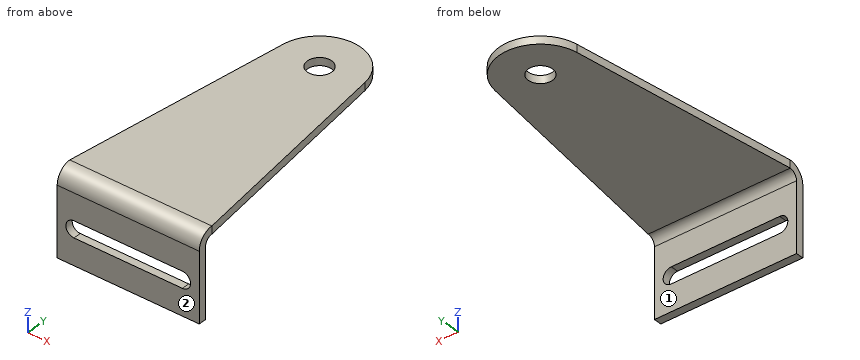
Autodesk Inventor part; units mm, degrees
ref_plane "YZ Plane" through (0, 0, 0) normal (1, 0, 0) x (0, 1, 0)
ref_plane "XZ Plane" through (0, 0, 0) normal (0, 1, 0) x (-1, 0, 0)
ref_plane "XY Plane" through (0, 0, 0) normal (0, 0, 1) x (1, 0, 0)
sketch "Boceto1" plane through (0, 0, 0) normal (0, 1, 0) x (-1, 0, 0)
  line L0 (-17.5, 8.5) -> (17.5, 8.5)
  line L1 (17.5, 8.5) -> (17.5, -8.5)
  line L2 (17.5, -8.5) -> (-17.5, -8.5)
  line L3 (-17.5, -8.5) -> (-17.5, 8.5)
  line L4 (-17.5, 8.5) -> (17.5, -8.5) construction
  line L5 (17.5, 8.5) -> (-17.5, -8.5) construction
  point P0 (0, 0)
  dimension "d0" = 35
  dimension "d1" = 17
extrude "Placa1" add sketch "Boceto1" along normal blind 1.91
sketch "Boceto2" plane through (17.5, 3.82, 10.41) normal (0, 0, 1) x (1, 0, 0)
  line L0 (-35, 0) -> (0, 0)
  line L1 (0, 0) -> (0, 66.18)
  line L2 (0, 66.18) -> (-35, 66.18)
  line L3 (-35, 66.18) -> (-35, 0)
edge flange "Pestaña1" height 70 angle 90 thickness 1.91 bend radius 1.91 thickness toward (0, 0, 1) relief tear relief width 1.91 relief depth 0.955 edges at (0, 1.91, 8.5) wall of the first edge with corners at (-17.5, 3.82, 10.41) (17.5, 3.82, 10.41) (17.5, 70, 10.41) (-17.5, 70, 10.41)
bend "Doblez1"
corner "Esquina1"
sketch "Boceto5" plane through (-17.5, 70, 12.32) normal (0, 0, 1) x (1, 0, 0)
  arc A0 (27.5986, -10.5074) -> (7.4014, -10.5074) centre (17.5, -11.85) ccw
  line L0 (0, -66.18) -> (7.4014, -10.5074)
  line L1 (35, -66.18) -> (27.5986, -10.5074)
  line L2 (0, 0) -> (35, 0)
  line L3 (0, -66.18) -> (0, 0)
  line L4 (0, 0) -> (35, 0)
  line L5 (35, 0) -> (35, -66.18)
  point P0 (17.5, -70)
  dimension "d21" = 20.375
extrude "Cortar2" cut sketch "Boceto5" against normal blind 1.91
sketch "Boceto6" plane through (-17.5, 3.82, 12.32) normal (0, 0, 1) x (1, 0, 0)
  line L0 (7.4014, 55.6726) -> (0, 0)
  line L1 (0, 0) -> (35, 0)
  line L2 (35, 0) -> (27.5986, 55.6726)
  arc A0 (27.5986, 55.6726) -> (7.4014, 55.6726) centre (17.5, 54.33) ccw
  circle A1 centre (17.5, 54.33) radius 3
  point P0 (17.5, -3.82)
  dimension "d26" = 6
extrude "Cortar3" cut sketch "Boceto6" against normal blind 1.91 contours A1
sketch "Boceto7" plane through (0, 1.91, 0) normal (0, 1, 0) x (1, 0, 0)
  line L0 (13.3569, 0) -> (-13.3569, 0) construction
  line L1 (13.3569, 2) -> (-13.3569, 2)
  line L2 (-13.3569, -2) -> (13.3569, -2)
  arc A0 (13.3569, -2) -> (13.3569, 2) centre (13.3569, 0) ccw
  arc A1 (-13.3569, 2) -> (-13.3569, -2) centre (-13.3569, 0) ccw
  point P0 (0, 0)
  dimension "d29" = 4
extrude "Cortar4" cut sketch "Boceto7" against normal blind 1.91
equation "\"d24\" = Grosor"
equation "\"d27\" = Grosor"
equation "\"d30\" = Grosor"
equation "\"d2\" = Grosor"
equation "\"d3\" = Anchura_desahogo_plegado"
equation "\"d4\" = Profundidad_desahogo_plegado"
equation "\"d5\" = Remanente_mínimo"
equation "\"d6\" = Radiodetransición"
equation "\"d9\" = Radio_pliegue"
equation "\"d10\" = Tamaño_destalonado"
equation "\"d11\" = TamañoSeparación"
equation "\"d12\" = Tamaño_de_radio_de_Jacobi"
equation "\"Radio_pliegue\" = Grosor"
equation "\"Anchura_desahogo_plegado\" = Grosor"
equation "\"Profundidad_desahogo_plegado\" = 0.5 * Grosor"
equation "\"Tamaño_destalonado\" = 4 * Grosor"
equation "\"Remanente_mínimo\" = 2 * Grosor"
equation "\"Radiodetransición\" = Radio_pliegue"
equation "\"Tamaño_de_radio_de_Jacobi\" = Radio_pliegue"
equation "\"TamañoSeparación\" = Grosor"
properties part number "soporte_barra" material "Acero AISI 1006 85 LC"
Can you work these out from the model? Positions are in its coordinate system, mm. Face numbers are marked on the shaded views. A direction names the side the tool comes from. Give positions to 0.01 mm unless a question says otherwise; leave off trailing zeros. Write each loop counter-clockwise with the first axis right and the second up, starting at its lowest first coordinate (ties: lowest second). Pieces come first, ordered by that corner, then holes. Notation, with made-up numbers: M -19.75,83.25 L -6.75,83.25 A21 cw -6.75,117.25 Z; hole C 56.25,11 d1. An arc over 180 degrees is marked long. Answer in a Markdown table with one row per item. Add a question column.
Item 1: Imagine slicing it at D-D, the plane y = 58.15. Write out the boundary of the cut face in (x, z), plus the area to 3 significant figures.
Item 2: Imagine slicing it at C-C, the plane x = 7. Write out the boundary of the cut face in (y, z).
Item 3: On a 3-axis mill with a long thin cutter (end or side, diameter ignored), from which of +Z, -Z, +X, -X, +Y, -Y can I reach the whole of each face in a straight line? I mean the marked faces 1 and 2. Say none if no direction works.
Item 4: Imagine slicing it at B-B, the plane z = 0. Write out the boundary of the cut face in (x, y).
Item 5: For pin 1 Ø2 at (x, y) = (-4.5, 0.5) entering from +Z; pin 2 Ø10.5 at (x, y) = (-1.5, 36.5) entering from -Z; pin 3 Ø3 at (x, z) = (-2, 2.5) entering from +Y, each with a flat end and sliding along its axis, tell me the tip position at first contact or that it passes through.
Item 6: Please list where these lines run through material, in increasing order: L1, parallel to Z at x = 0, y = 40.5; L2, parallel to Y at x = -5.5, z = -4.75; L3, parallel to Y at x = 0, z = 11.6.
Item 7: Imagine slicing it at A-A, the plane x = 0. Write out the boundary of the cut face in (y, z).
Evaluation:
| question | item | result |
|---|---|---|
| 1 | outline | M -10.28,10.41 L -3,10.41 L -3,12.32 L -10.28,12.32 Z; M 3,10.41 L 10.28,10.41 L 10.28,12.32 L 3,12.32 Z |
| 1 | area | 27.8 mm² |
| 2 | outline | M 0,-8.5 L 1.91,-8.5 L 1.91,-2 L 0,-2 Z; M 0,2 L 1.91,2 L 1.91,8.5 A1.91 cw 3.82,10.41 L 65.55,10.41 L 65.55,12.32 L 3.82,12.32 A3.82 ccw 0,8.5 Z |
| 3 | face 1 | -Z, +X, -X, +Y |
| 3 | face 2 | +Z, -Z, +X, -X, -Y |
| 4 | outline | M -17.5,0 L -15.36,0 L -15.36,1.91 L -17.5,1.91 Z; M 15.36,0 L 17.5,0 L 17.5,1.91 L 15.36,1.91 Z |
| 5 | pin 1 | stops at z = 11.53 |
| 5 | pin 2 | stops at z = 10.41 |
| 5 | pin 3 | stops at y = 1.91 |
| 6 | L1 | z = 10.41 to 12.32 |
| 6 | L2 | y = 0 to 1.91 |
| 6 | L3 | y = 1.59 to 55.15, 61.15 to 68.34 |
| 7 | outline | M 0,-8.5 L 1.91,-8.5 L 1.91,-2 L 0,-2 Z; M 0,2 L 1.91,2 L 1.91,8.5 A1.91 cw 3.82,10.41 L 55.15,10.41 L 55.15,12.32 L 3.82,12.32 A3.82 ccw 0,8.5 Z; M 61.15,10.41 L 68.34,10.41 L 68.34,12.32 L 61.15,12.32 Z |
